Verification items for this drawing (mm, ordinates from the low corner). Coordinates: 2 decimals unless noted, no trailing zeros. Loops run counter-clockwise (first coordinate to the right, second up) from the corner with the lowest first, then second, coordinate; pieces in that order, holes last. Notation, with made-up numbers: M 38,34 L 94,34 A16 ccw 94,59 Z; hole C 3.25,7 d1. An arc over 180 degrees is marked long. Return JSON: item names as keys, results as strings.
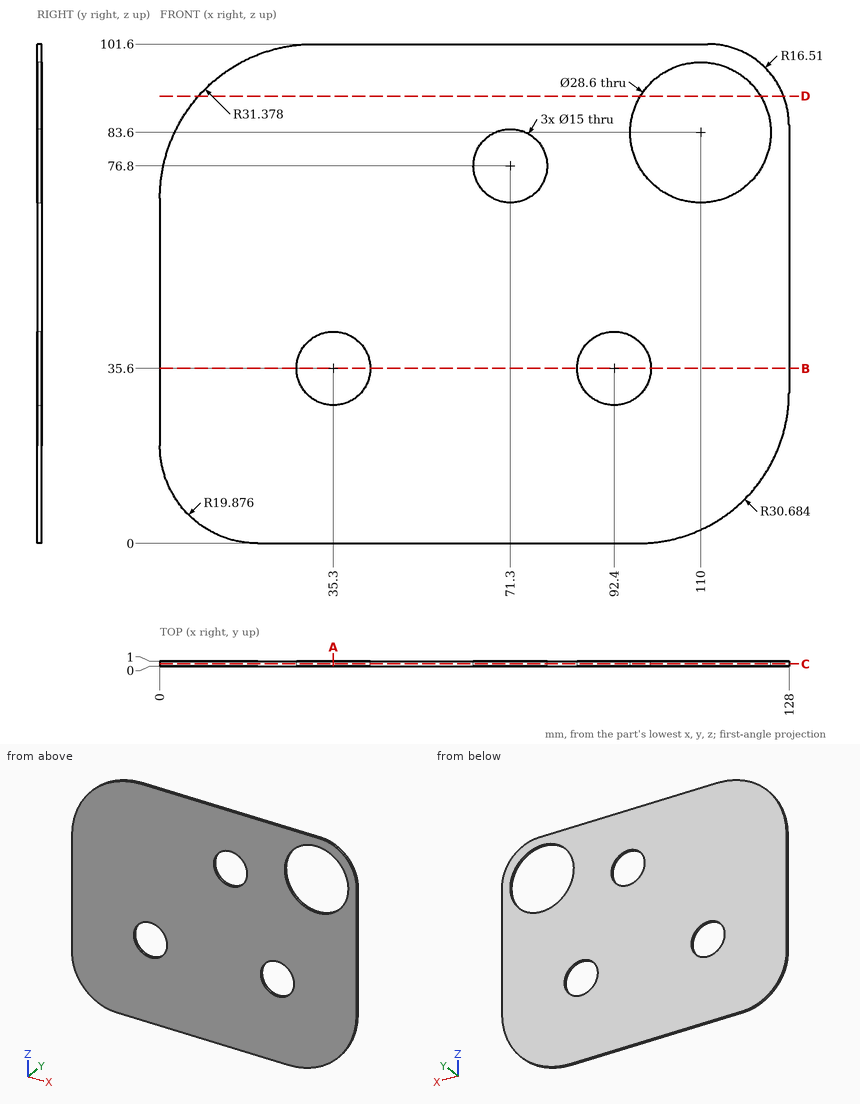
1) Section check D-D on z = 91. Record the cut outline in (x, y) (1 decimal).
Answers:
{"outline": "M 7.9,0 L 97.8,0 L 97.8,1 L 7.9,1 Z; M 122.2,0 L 126.9,0 L 126.9,1 L 122.2,1 Z"}
2) Section check A-A on x = 35.3. Record the cut outline in (y, z).
Answers:
{"outline": "M 0,0 L 1,0 L 1,28.1 L 0,28.1 Z; M 0,43.1 L 1,43.1 L 1,101.6 L 0,101.6 Z"}
3) Section check C-C on y = 0.5. Record the cut outline in (x, z) (1 decimal).
Answers:
{"outline": "M 0,19.9 A19.9 ccw 19.9,0 L 97.3,0 A30.7 ccw 128,30.7 L 128,85.1 A16.5 ccw 111.5,101.6 L 31.4,101.6 A31.4 ccw 0,70.2 Z; hole C 35.3,35.6 d15; hole C 71.3,76.8 d15; hole C 92.4,35.6 d15; hole C 110,83.6 d28.6"}
4) Scan lines: line 1 along X through (y, z) = (0.5, 71.5) (1 decimal); line 2 along X through (y, z) = (0.55, 76.8); line 3 along X through (y, z) = (0.3, 95) (1 decimal). Record each from-to range of solid material in increasing order. Write a range as [from, to].
Answers:
{"line 1": "[0, 66], [76.6, 102.4], [117.6, 128]", "line 2": "[0.7, 63.8], [78.8, 97.42], [122.58, 128]", "line 3": "[12.1, 101.4], [118.6, 124.7]"}
5) Section check B-B on z = 35.6. Record the cut outline in (x, y).
Answers:
{"outline": "M 0,0 L 27.8,0 L 27.8,1 L 0,1 Z; M 42.8,0 L 84.9,0 L 84.9,1 L 42.8,1 Z; M 99.9,0 L 128,0 L 128,1 L 99.9,1 Z"}
